The model under review builds one solid part; all positions refer to its coordinate system, in mm. Face numbers are marked on the shaded views. Round coordinates to 2 decimals unless told otherwise and drop trailing zeros. Order: outer loops, then holes, each group sorted by start corner. A loop starts at its lowest first (then second) coordinate and runs counter-clockwise, first axis right, second up. Notation, with made-up numbers: M -2,-19.5 L 9,-19.5 A23 cw 9,14.5 Z; hole C 86.25,88 d11. An arc over 180 degrees is marked long. Use a Markdown table: item, result. Add a question column.
1. The part is to be moulded in two halves that separate along X. For the marked faces 1 and 2, say which applies: +X half, -X half, draft (parallel to the pull), parting line (faces both ways), or undercut.
2. To check wall thickness, follow probe 1 along Z at (x, y) = (-73, 2.15); probe 2 along X at (y, z) = (2.65, -13.75); probe 3 along X at (y, z) = (1.5, -20). State the ranges of each line that lie inside material, in increasing order.
3. Insertion check: P1, Ø1, axis at y = 1, z = -18.5, coming from the +X side. The pin has a flat end and moves straight along its axis. Give the tip position at first contact, or say it passes through.
4. Consider section A-A on x = -71. State the section outline as (y, z) points.
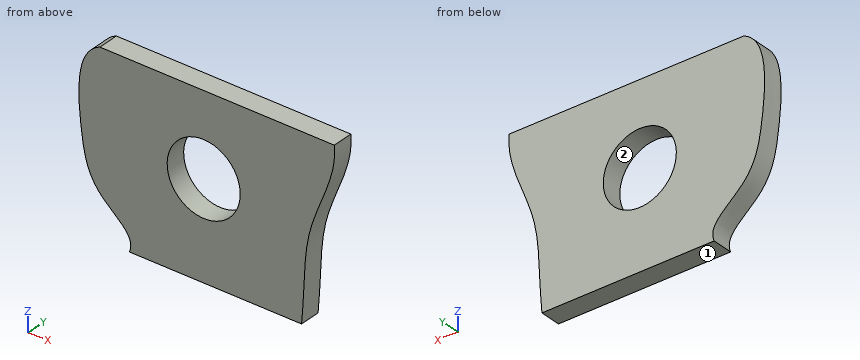
from build123d import *

# Parameters (mm, degrees)
DODANIE_WYCI_GNI_CIE1_DEPTH = 3
SZKIC2_R                    = 5.25
WYTNIJ_WYCI_GNI_CIE1_DEPTH  = 123.478678077
SZKIC3_W                    = 83.042343976
SZKIC3_H                    = 22.425434336
SZKIC3_W_2                  = 92.40199983
SZKIC3_H_2                  = 23.262955651
WYTNIJ_WYCI_GNI_CIE2_DEPTH  = 123.478678077
WYTNIJ_WYCI_GNI_CIE3_DEPTH  = 114.371150202


with BuildPart() as part:
    # Szkic1 → Dodanie-wyciągnięcie1 (new body)
    with BuildSketch(Plane(origin=(0, 0, 0), x_dir=(1, 0, 0), z_dir=(0, 1, 0))):
        with BuildLine():
            Line((-97.678150888, 49.4149367), (-32.744802343, 49.4149367))
            add(Edge.make_bspline(
                [(-32.744802343, 49.4149367), (-29.306315805, 38.482449345), (-35.086079974, 19.443677378), (-46.815707035, -0.452000217), (-49.516641207, -11.467220133), (-49.715376383, -12.36868324)],
                knots=[0.154589074, 0.154589074, 0.154589074, 0.154589074, 0.39168588, 0.61157723, 0.631041789, 0.631041789, 0.631041789, 0.631041789], degree=3))
            Line((-49.715376383, -12.36868324), (-112.027633116, -12.36868324))
            add(Edge.make_bspline(
                [(-97.678150888, 49.4149367), (-95.996907517, 42.817556452), (-98.213660437, 28.328196325), (-109.215623339, 9.191600555), (-111.919105273, -6.718294499), (-112.027633116, -12.36868324)],
                knots=[0.127638687, 0.127638687, 0.127638687, 0.127638687, 0.284871496, 0.500245721, 0.624008673, 0.624008673, 0.624008673, 0.624008673], degree=3))
        make_face()
    extrude(amount=DODANIE_WYCI_GNI_CIE1_DEPTH)

    # Szkic2 → Wytnij-wyciągnięcie1 (cut, through all)
    with BuildSketch(Plane(origin=(0, 3, 0), x_dir=(1, 0, 0), z_dir=(0, 1, 0))):
        with Locations(Location((-73.202778656, 17.886796147, 0), (0, 0, 270))):
            Circle(SZKIC2_R)
    extrude(amount=-WYTNIJ_WYCI_GNI_CIE1_DEPTH, mode=Mode.SUBTRACT)

    # Szkic3 → Wytnij-wyciągnięcie2 (cut, through all)
    with BuildSketch(Plane(origin=(0, 3, 0), x_dir=(1, 0, 0), z_dir=(0, 1, 0))):
        with Locations((-62.244564273, 42.931839176)):
            Rectangle(SZKIC3_W, SZKIC3_H)
        with Locations((-68.037284909, -5.510245727)):
            Rectangle(SZKIC3_W_2, SZKIC3_H_2)
    extrude(amount=-WYTNIJ_WYCI_GNI_CIE2_DEPTH, mode=Mode.SUBTRACT)

    # Szkic4 → Wytnij-wyciągnięcie3 (cut, through all)
    with BuildSketch(Plane(origin=(0, 3, 0), x_dir=(1, 0, 0), z_dir=(0, 1, 0))):
        with BuildLine():
            add(Edge.make_bspline(
                [(-88.689938792, 36.010164682), (-86.071156922, 34.618848613), (-81.089784858, 30.465171833), (-89.644619421, 25.502930729), (-91.094282475, 17.320923853), (-91.890518911, 4.656814481), (-70.345884336, 7.408238477), (-112.625080918, -8.466168712), (-128.254843762, 14.531836441), (-112.47359997, 31.235119166), (-98.588015331, 41.268851209), (-88.689938792, 36.010164682)],
                knots=[0, 0, 0, 0, 0.056310149, 0.105139867, 0.166932459, 0.258637906, 0.305170294, 0.520996128, 0.678649021, 0.787167396, 1, 1, 1, 1], degree=3))
        make_face()
        with BuildLine():
            add(Edge.make_bspline(
                [(-58.506782582, 38.587883821), (-59.676552515, 36.005094764), (-58.575510558, 28.258639934), (-58.925436397, 17.111965112), (-49.705448185, 4.127794868), (-72.040088465, -9.964706752), (-44.500598429, -4.631349285), (-29.373358451, 0.777563949), (-22.973161664, 21.590397636), (-30.322336493, 42.955036515), (-55.380407315, 45.490752157), (-58.506782582, 38.587883821)],
                knots=[0, 0, 0, 0, 0.066886355, 0.137581529, 0.239375905, 0.330501418, 0.448637218, 0.557955025, 0.707331232, 0.821236773, 1, 1, 1, 1], degree=3))
        make_face()
    extrude(amount=-WYTNIJ_WYCI_GNI_CIE3_DEPTH, mode=Mode.SUBTRACT)


solid = part.part
Answer block:
| question | item | result |
|---|---|---|
| 1 | face 1 | draft |
| 1 | face 2 | undercut |
| 2 | probe 1 | -31.72 to -23.13, -12.64 to -6.12 |
| 2 | probe 2 | -91.14 to -76.44, -69.97 to -56.08 |
| 2 | probe 3 | -90.52 to -78.01, -68.4 to -58.19 |
| 3 | P1 | x = -57.68 |
| 4 | outline | M 0,-31.72 L 3,-31.72 L 3,-22.65 L 0,-22.65 Z; M 0,-13.12 L 3,-13.12 L 3,-6.12 L 0,-6.12 Z |
